```python
from build123d import *

# Parameters (mm, degrees)
SKETCH2_R           = 12.7
BOSS_EXTRUDE1_DEPTH = 12.7
CUT_EXTRUDE1_DEPTH  = 22.997045256


with BuildPart() as part:
    # Sketch2 → Boss-Extrude1 (new body)
    with BuildSketch(Plane(origin=(0, 0, 0), x_dir=(0, 1, 0), z_dir=(0, 0, 1))):
        with Locations(Location((0, 0, 0), (0, 0, 270))):
            Circle(SKETCH2_R)
    extrude(amount=BOSS_EXTRUDE1_DEPTH)

    # Sketch3 → Cut-Extrude1 (cut, through all)
    with BuildSketch(Plane.XY.offset(12.7)):
        Polygon((-2.492998462, -4.318), (2.492998462, -4.318), (4.985996925, 0), (2.492998462, 4.318), (-2.492998462, 4.318), (-4.985996925, 0), align=None)
    extrude(amount=-CUT_EXTRUDE1_DEPTH, mode=Mode.SUBTRACT)


solid = part.part
```
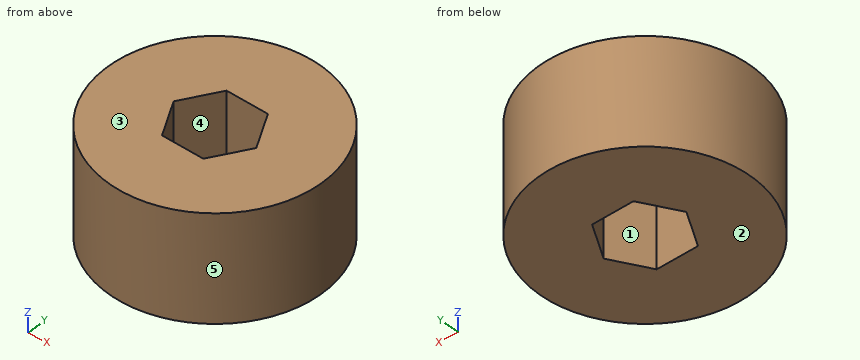
Model file for the job. Use its own axes, mm. Face numbers are marked on the shaded views. A direction names the side the tool comes from. Coordinates: 2 decimals unless noted, no trailing zeros. Write each loop counter-clockwise with the first axis right and the second up, starting at its lowest first coordinate (ties: lowest second). Pieces come first, ordered by that corner, then holes. Notation, with made-up numbers: (50.5, 56) - (74.5, 56) arc R34 cw to (74.5, 87) - close; hole circle Ø10 at (44, -33). An arc over 180 degrees is marked (long way). One line per question, with ' | ' between items. Start each with the question number.
Q1. Cut at D-D, the plane x = -6. List the corners of the cut face in (y, z), then the cut area to 3 significant figures.
Q2. Pin check, flat tips, straight feed: pin 1 (5.5 mm diameter, centred on x = -0.5, z = 7, fed in from +Y); pin 2 (5 mm diameter, centred on x = 4, z = 11, fed in from -Y); pin 3 (5 mm diameter, centred on x = -7, z = 4, fed in from -Y). Stop position of each tip, or through.
Q3. Cut at C-C, the plane y = 9.25. List the corners of the cut face in (x, z), then the cut area to 3 significant figures.
Q4. Drill centre lines: line 1 (Y direction, x = 0, z = 2.5); line 2 (X direction, y = -1, z = 7.25); line 3 (X direction, y = 3.5, z = 2.25). Where is each one in solid material? Low to high. Write a range as [from, to].
Q5. Pull direction Y, two halves, no side cores. Call the marked faces 3, 4 and 5: pulls with the +Y half, pulls with the -Y half, needs draft (parallel to the pull), parting line crosses it, or undercut.
Q6. 3-axis set-ups, long thin cutter, end or side, ignore diameter. For the marked faces 1 and 2: which of +Z, -Z, +X, -X, +Y, -Y reach the whole face in a straight line?
Q7. Cut at A-A, the plane x = 0. List the corners of the cut face in (y, z).
Q8. Cut at B-B, the plane z = 4. List the corners of the cut face in (x, y), then the cut area to 3 significant figures.
Answer below:
1) outline: (-11.19, 0) - (11.19, 0) - (11.19, 12.7) - (-11.19, 12.7) - close | area: 284 mm^2
2) pin 1: y = 12.7 | pin 2: y = -12.61 | pin 3: y = -11.88
3) outline: (-8.7, 0) - (8.7, 0) - (8.7, 12.7) - (-8.7, 12.7) - close | area: 221 mm^2
4) line 1: [-12.7, -4.32], [4.32, 12.7] | line 2: [-12.66, -4.41], [4.41, 12.66] | line 3: [-12.21, -2.97], [2.97, 12.21]
5) face 3: needs draft | face 4: undercut | face 5: parting line crosses it
6) face 1: +Z, -Z | face 2: -Z, +X, -X, +Y, -Y
7) outline: (-12.7, 0) - (-4.32, 0) - (-4.32, 12.7) - (-12.7, 12.7) - close; (4.32, 0) - (12.7, 0) - (12.7, 12.7) - (4.32, 12.7) - close
8) outline: circle Ø25.4 at (0, 0); hole (-4.99, 0) - (-2.49, -4.32) - (2.49, -4.32) - (4.99, 0) - (2.49, 4.32) - (-2.49, 4.32) - close | area: 442 mm^2
